Autodesk Inventor part; units mm, degrees
ref_plane "YZ Plane" through (0, 0, 0) normal (1, 0, 0) x (0, 1, 0)
ref_plane "XZ Plane" through (0, 0, 0) normal (0, 1, 0) x (-1, 0, 0)
ref_plane "XY Plane" through (0, 0, 0) normal (0, 0, 1) x (1, 0, 0)
sketch "Sketch1" plane through (0, 0, 0) normal (0, 0, 1) x (1, 0, 0)
  line L0 (-11.7228, 9.8454) -> (238.2772, 9.8454)
  line L1 (238.2772, 9.8454) -> (238.2772, -340.1546)
  line L2 (238.2772, -340.1546) -> (-11.7228, -340.1546)
  line L3 (-11.7228, -340.1546) -> (-11.7228, 9.8454)
  point P0 (0, 0)
  dimension "d0" = 250
  dimension "d1" = 350
extrude "Extrusion1" add sketch "Sketch1" along normal blind 15
sketch "Sketch2" plane through (0, 0, 15) normal (0, 0, 1) x (1, 0, 0)
  line L0 (-11.7228, 9.8454) -> (-11.7228, -340.1546)
  line L1 (238.2772, -340.1546) -> (238.2772, 9.8454)
  line L2 (-11.7228, -70.1546) -> (238.2772, -70.1546)
  line L3 (238.2772, -70.1546) -> (238.2772, -170.1546)
  line L4 (238.2772, -170.1546) -> (-11.7228, -170.1546)
  line L5 (-11.7228, -170.1546) -> (-11.7228, -70.1546)
  line L6 (238.2772, 9.8454) -> (-11.7228, 9.8454)
  line L7 (-11.7228, -340.1546) -> (238.2772, -340.1546)
  point P0 (0, 0)
  point P1 (-11.7228, -170.1546)
  dimension "d4" = 80
  dimension "d5" = 170
extrude "Extrusion2" add sketch "Sketch2" along normal blind 10 contours L2 L1 L4 L0
sketch "Sketch3" plane through (0, 0, 25) normal (0, 0, 1) x (1, 0, 0)
  point P0 (0, 0)
  point P1 (43.9699, -124.4167)
  point P2 (136.2084, -123.6085)
hole "Hole1" at (43.9699, -124.4167, 25) at (136.2084, -123.6085, 25) direction (0, 0, -1) diameter 25.4 end through all
properties part number "base"
For this review, take the finished solid that the model builds, in its own axes (mm). A direction names the side the tool comes from. Round coordinates to 2 decimals unless told otherwise and drop trailing zeros. Write each loop counter-clockwise with the first axis right and the second up, starting at its lowest first coordinate (ties: lowest second). Pieces come first, ordered by that corner, then holes. Notation, with made-up numbers: (70.5, 16.25) -> (112.5, 16.25) arc R20 ccw to (112.5, 52.25) -> close; hole circle Ø1 at (6, -0.75). An arc over 180 degrees is marked (long way). Use one line per item in the form item = value.
Q1. The part is to be moulded in two halves that separate along Y. For faces 1 (the flat face through (-11.723, -168, 10)), 2 (the cylindrical face through (125.5, -130.44, 12.32)), 3 (the flat face through (115, -340.155, 7)), say which applies: released by +Y, released by -Y, zero draft, split by the parting line, or undercut.
Resolved:
face_1 = zero draft
face_2 = undercut
face_3 = released by -Y
Q2. Machinability: for faces 4 (the flat face through (238.277, -163, 10)), 5 (the flat face through (112, -254, 15)), 6 (the flat face through (112, -70.155, 20)), which of the approach directions +Z, -Z, +X, -X, +Y, -Y give a long, thin tool a straight path to every point of the face, cutting with its end or side? Answer none if there is none.
Resolved:
face_4 = +Z, -Z, +X, +Y, -Y
face_5 = +Z, +X, -X, -Y
face_6 = +Z, +X, -X, +Y
Q3. Clearance check with flat-ended pins moving along their axes: pin 1 Ø5 at (x, z) = (151, 22) entering from +Y; pin 2 Ø1 at (x, z) = (125.5, 17.5) entering from -Y; pin 3 Ø10 at (x, y) = (35.5, -247.5) entering from +Z. State where each tip first meets the part, or that it passes through.
Resolved:
pin_1 = -70.15
pin_2 = -170.15
pin_3 = 15
Q4. Consider section C-C (z = 19.5). State the section outline as (x, y) points.
Resolved:
outline = (-11.72, -170.15) -> (238.28, -170.15) -> (238.28, -70.15) -> (-11.72, -70.15) -> close; hole circle Ø25.4 at (43.97, -124.42); hole circle Ø25.4 at (136.21, -123.61)
Q5. To check wall thickness, follow probe 1 along Z at (x, y) = (70, -217.5); probe 2 along Y at (x, z) = (186.5, 20.5); probe 3 along Y at (x, z) = (43.5, 23.25). State the ranges of each line that lie inside material, in increasing order. Write a range as from..to.
Resolved:
probe_1 = 0..15
probe_2 = -170.15..-70.15
probe_3 = -170.15..-137.11, -111.73..-70.15
Q6. Consider section B-B (y = -204.5). State the section outline as (x, z) points.
Resolved:
outline = (-11.72, 0) -> (238.28, 0) -> (238.28, 15) -> (-11.72, 15) -> close
Q7. Consider section A-A (x = 166). State the section outline as (y, z) points.
Resolved:
outline = (-340.15, 0) -> (9.85, 0) -> (9.85, 15) -> (-70.15, 15) -> (-70.15, 25) -> (-170.15, 25) -> (-170.15, 15) -> (-340.15, 15) -> close
